Check sheet for the modelled part. Datum: model origin and axes. Units: mm. Face numbers are marked on the shaded views. A direction names the side the tool comes from. Round coordinates to 2 decimals unless told otherwise and drop trailing zeros. Loops run counter-clockwise (first coordinate to the right, second up) from the corner with the lowest first, then second, coordinate; pieces in that order, holes last. Notation, with made-up numbers: (70.25, 20) -> (90.25, 20) arc R15 ccw to (90.25, 24) -> close; hole circle Ø9 at (60.5, 10). An arc over 180 degrees is marked (long way). One line per item, written item: value. Start each with the question number.
1. Release check for a two-part mould opening along Z. For the marked faces 1, 2 and 3 record: +Z half, -Z half, draft (parallel to the pull), parting line (faces both ways), or undercut.
2. Material ranges on L1, parallel to Z at x = -10, y = -3; L2, parallel to Y at x = -13.5, z = 4.75; L3, parallel to X at y = -9.5, z = 3.25, recorded low to high.
3. Cross-section at B-B on x = -10. Record the cut outline in (y, z).
4. Cross-section at C-C on x = -12.25. Record the cut outline in (y, z), then the cut area to 3 significant figures.
5. Cross-section at D-D on y = -4.5. Record the cut outline in (x, z).
6. Cross-section at A-A on z = 5. Record the cut outline in (x, y), then the cut area to 3 significant figures.
7. Go/stop test with flat-tipped pins: pin 1 (1.2 mm diameter, centred on x = -7.5, y = -11, fed in from +Z); pin 2 (3 mm diameter, centred on x = -5.5, z = 8.5, fed in from -Y). Record where each tip stops, or that it passes through.
8. Set-up check for the marked faces 4 and 5: record each of +Z, -Z, +X, -X, +Y, -Y from which the full face is reachable in a straight line by a thin tool's end or side.
from build123d import *

# Parameters (mm, degrees)
F0_W     = 15
F0_H     = 12.5
F1_DEPTH = 12.5
F2_SIZE2 = 5.0588138763
F2_SIZE  = 7.5
F3_W     = 2.5
F3_H     = 10
F4_DEPTH = 15.001
F5_R     = 2
F6_DEPTH = 10.001


with BuildPart() as f1:
    # F0 (on Front) → F1 (new body)
    with BuildSketch(Plane.XZ):
        with Locations((-7.5, 6.25)):
            Rectangle(F0_W, F0_H)
    extrude(amount=F1_DEPTH)

    # F2
    f2_edges = [f1.edges().sort_by_distance(p)[0] for p in [
        (0, -6.25, 12.5),
    ]]
    f2_side = f1.faces().sort_by_distance((-7.5, -6.25, 12.5))[0]
    chamfer(f2_edges, length=F2_SIZE, length2=F2_SIZE2, reference=f2_side)

    # F3 (on face) → F4 (cut, through all)
    with BuildSketch(Plane.YZ):
        with Locations((-11.25, 7.5)):
            Rectangle(F3_W, F3_H)
    extrude(amount=-F4_DEPTH, mode=Mode.SUBTRACT)

    # F5 (on face) → F6 (cut, through all)
    with BuildSketch(Plane.XZ.offset(10)):
        with Locations((-10, 5)):
            Circle(F5_R)
    extrude(amount=-F6_DEPTH, mode=Mode.SUBTRACT)


solid = f1.part
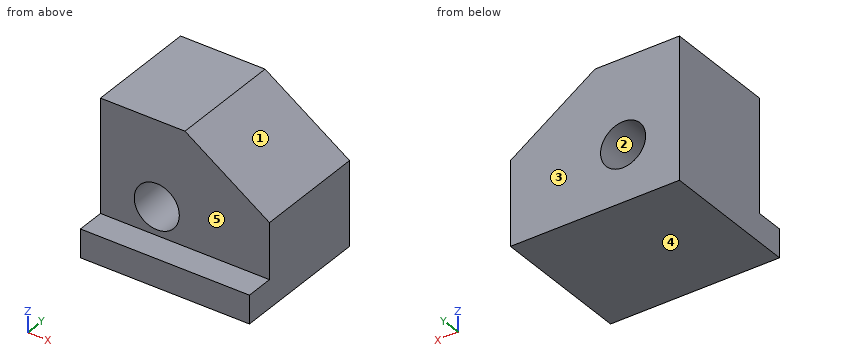
Taken from the geometry:
1. face 1: +Z half
1. face 2: undercut
1. face 3: draft
2. L1: z = 0 to 3, 7 to 12.5
2. L2: y = -10 to 0
2. L3: x = -15 to -10.97, -9.03 to 0
3. outline: (-12.5, 0) -> (0, 0) -> (0, 3) -> (-10, 3) -> (-10, 2.5) -> (-12.5, 2.5) -> close; (-10, 7) -> (0, 7) -> (0, 12.5) -> (-10, 12.5) -> close
4. outline: (-12.5, 0) -> (0, 0) -> (0, 12.5) -> (-10, 12.5) -> (-10, 2.5) -> (-12.5, 2.5) -> close
4. area: 131 mm2
5. outline: (-15, 0) -> (0, 0) -> (0, 7.44) -> (-7.5, 12.5) -> (-15, 12.5) -> close; hole circle Ø4 at (-10, 5)
6. outline: (-15, -10) -> (-12, -10) -> (-12, 0) -> (-15, 0) -> close; (-8, -10) -> (0, -10) -> (0, 0) -> (-8, 0) -> close
6. area: 110 mm2
7. pin 1: stops at z = 2.5
7. pin 2: stops at y = -10
8. face 4: -Z, +X, -X, +Y, -Y
8. face 5: +Z, +X, -X, -Y
